Autodesk Inventor part; units mm, degrees
ref_plane "YZ Plane" through (0, 0, 0) normal (1, 0, 0) x (0, 1, 0)
ref_plane "XZ Plane" through (0, 0, 0) normal (0, 1, 0) x (-1, 0, 0)
ref_plane "XY Plane" through (0, 0, 0) normal (0, 0, 1) x (1, 0, 0)
sketch "Esquisse1" plane through (0, 0, 0) normal (0, 1, 0) x (-1, 0, 0)
  line L0 (0, 0) -> (12, 0)
  line L1 (12, 0) -> (12, -10)
  line L2 (12, -10) -> (0, -10)
  line L3 (0, -10) -> (0, 0)
  dimension "d0" = 10
  dimension "d1" = 12
extrude "Extrusion1" add sketch "Esquisse1" along normal blind 22.4
sketch "Esquisse2" plane through (0, 22.4, 0) normal (0, 1, 0) x (1, 0, 0)
  line L0 (-12, 0) -> (0, 0) construction
  line L1 (0, 0) -> (0, 10) construction
  line L2 (0, 10) -> (-12, 10) construction
  line L3 (-12, 10) -> (-12, 0) construction
  line L4 (-12, 5) -> (0, 5) construction
  line L5 (0, 0) -> (0, 10) construction
  circle A0 centre (-6, 5) radius 1.5
  dimension "d4" = 3
extrude "Extrusion2" add sketch "Esquisse2" along normal blind 9
sketch "Esquisse3" plane through (0, 0, 0) normal (0, -1, 0) x (1, 0, 0)
  line L0 (0, 0) -> (-12, 0) construction
  line L1 (-12, 0) -> (-12, -10) construction
  line L2 (-12, -10) -> (0, -10) construction
  line L3 (0, -10) -> (0, 0) construction
  line L4 (0, -10) -> (-12, -10)
  line L5 (-12, -10) -> (-12, 7)
  line L6 (-12, 7) -> (0, 7)
  line L7 (0, 7) -> (0, -10)
  line L8 (-12, 0) -> (-12, -10)
  dimension "d7" = 17
extrude "Extrusion3" add sketch "Esquisse3" along normal blind 6.4
properties part number "motor"
Check sheet for the modelled part. Datum: model origin and axes. Units: mm. A direction names the side the tool comes from. Round coordinates to 2 decimals unless told otherwise and drop trailing zeros. Loops run counter-clockwise (first coordinate to the right, second up) from the corner with the lowest first, then second, coordinate; pieces in that order, holes last.
1. Mould release check, pull along Y, two halves, no side actions. Record for faces 1 (the flat face through (-12, 5, -4)), 2 (the flat face through (-6, -6.4, -1)), 3 (the flat face through (-4.6, 22.4, -3.8)): released by +Y, released by -Y, zero draft, split by the parting line, or undercut.
2. Scan lines: probe 1 along Z at (x, y) = (-4.75, 11.5); probe 2 along Y at (x, z) = (-9, 0.5); probe 3 along Y at (x, z) = (-6.25, -1). Record each from-to range of solid material in increasing order.
3. Set-up check for faces 4 (the cylindrical face through (-7.11, 26.84, -3.99)), 5 (the flat face through (-6, 31.4, -5)), 6 (the flat face through (-6, 11, 0)): record each of +Z, -Z, +X, -X, +Y, -Y from which the full face is reachable in a straight line by a thin tool's end or side.
4. Sectioned sample at C-C on y = 22. Record the boundary of the cut face in (x, z), and give its area (3 significant figures).
5. Sectioned sample at D-D on x = -1.5. Record the boundary of the cut face in (y, z), and give its area (3 significant figures).
6. Sectioned sample at A-A on z = -5. Record the boundary of the cut face in (x, y), and give its area (3 significant figures).
7. Gauge pin test, flat ends, axial feed: pin 1 Ø5.5 at (x, z) = (-7.5, 2.5) entering from +Y; pin 2 Ø1.5 at (x, z) = (-5.5, 3.5) entering from +Y; pin 3 Ø5 at (x, y) = (-4.5, 7.5) entering from +Z. Record the tip position at first contact, or that the pin passes through.
8. Sectioned sample at B-B on x = -6. Record the boundary of the cut face in (y, z).
Recorded:
1. face 1: zero draft
1. face 2: released by -Y
1. face 3: released by +Y
2. probe 1: z = -10 to 0
2. probe 2: y = -6.4 to 0
2. probe 3: y = -6.4 to 22.4
3. face 4: +Y
3. face 5: +Z, -Z, +X, -X, +Y
3. face 6: +Z, +X, -X, +Y
4. outline: (-12, -10) - (0, -10) - (0, 0) - (-12, 0) - close
4. area: 120 mm2
5. outline: (-6.4, -10) - (22.4, -10) - (22.4, 0) - (0, 0) - (0, 7) - (-6.4, 7) - close
5. area: 333 mm2
6. outline: (-12, -6.4) - (0, -6.4) - (0, 22.4) - (-4.5, 22.4) - (-4.5, 31.4) - (-7.5, 31.4) - (-7.5, 22.4) - (-12, 22.4) - close
6. area: 373 mm2
7. pin 1: stops at y = 22.4
7. pin 2: stops at y = 0
7. pin 3: stops at z = 0
8. outline: (-6.4, -10) - (22.4, -10) - (22.4, -6.5) - (31.4, -6.5) - (31.4, -3.5) - (22.4, -3.5) - (22.4, 0) - (0, 0) - (0, 7) - (-6.4, 7) - close
